Study the drawing (mm; zero at the part's minimum x, y, z) and answer. Coordinates: 2 decimals unless noted, no trailing zeros. Write each loop counter-clockwise with the first axis right and the second up, starting at its lowest first coordinate (ties: lowest second). Pieces come first, ordered by that corner, then holes. Notation, with made-up numbers: (-33, -6) -> (-11, -6) arc R27 ccw to (-11, 12) -> close; hole circle Ø9 at (-29, 22.25). An arc over 180 degrees is marked (long way). Write item = value, one per line. Start each with the question number.
1) Section A-A (y = 30) is taken. Determine the outline of the cut face in (x, z).
2) Section C-C (z = 1.6) is taken. Determine the outline of the cut face in (x, y).
3) Find the intervals of material crossed by line 1 along Y through (x, z) = (12, 0.4); line 2 along X through (y, z) = (33, 2.7); line 3 along Y through (x, z) = (24.5, 2.6), in increasing order. Write a range as from..to.
4) A flat-ended cylindrical pin translates along its axis: pin 1 Ø8 at (x, y) = (12, 37) entering from +Z. Find the tip coordinate at first contact, or state that the pin passes through.
5) Section B-B (x = 13) is taken. Determine the outline of the cut face in (y, z).
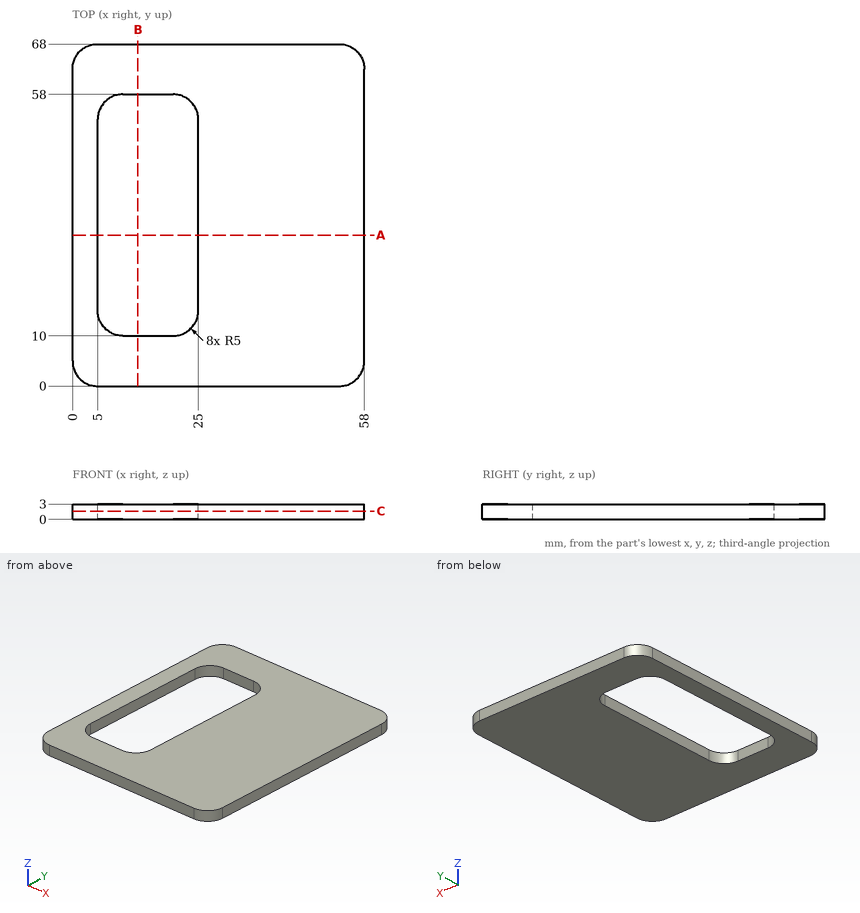
Answer key:
q1.outline = (0, 0) -> (5, 0) -> (5, 3) -> (0, 3) -> close; (25, 0) -> (58, 0) -> (58, 3) -> (25, 3) -> close
q2.outline = (0, 5) arc R5 ccw to (5, 0) -> (53, 0) arc R5 ccw to (58, 5) -> (58, 63) arc R5 ccw to (53, 68) -> (5, 68) arc R5 ccw to (0, 63) -> close; hole (5, 15) arc R5 ccw to (10, 10) -> (20, 10) arc R5 ccw to (25, 15) -> (25, 53) arc R5 ccw to (20, 58) -> (10, 58) arc R5 ccw to (5, 53) -> close
q3.line_1 = 0..10, 58..68
q3.line_2 = 0..5, 25..58
q3.line_3 = 0..12.82, 55.18..68
q4.pin_1 = through
q5.outline = (0, 0) -> (10, 0) -> (10, 3) -> (0, 3) -> close; (58, 0) -> (68, 0) -> (68, 3) -> (58, 3) -> close
